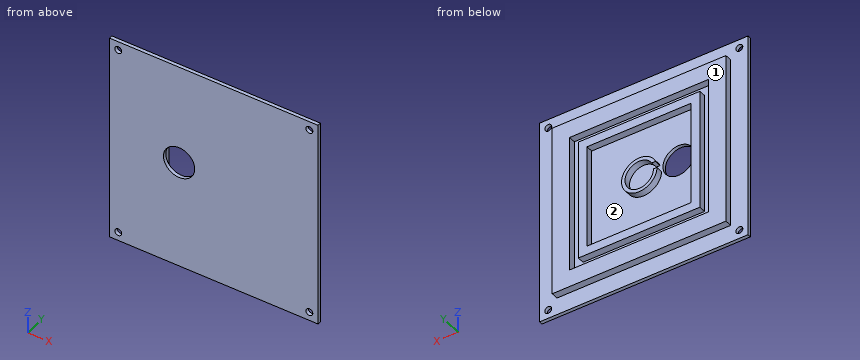
```python
from build123d import *

# Parameters (mm, degrees)
SKETCH1_W           = 152.4
SKETCH1_H           = 152.4
BOSS_EXTRUDE1_DEPTH = 2.54
SKETCH2_W           = 127
SKETCH2_H           = 127
BOSS_EXTRUDE3_DEPTH = 5.08
SKETCH3_W           = 101.6
SKETCH3_H           = 101.6
CUT_EXTRUDE2_DEPTH  = 5.08
SKETCH5_W           = 88.9
SKETCH5_H           = 88.9
BOSS_EXTRUDE4_DEPTH = 5.08
SKETCH6_W           = 76.2
SKETCH6_H           = 76.2
CUT_EXTRUDE3_DEPTH  = 5.08
BOSS_EXTRUDE5_DEPTH = 2.794
SKETCH8_R           = 11.43
CUT_EXTRUDE4_DEPTH  = 3.54
SKETCH9_R           = 2.54
CUT_EXTRUDE5_DEPTH  = 3.54
BOSS_EXTRUDE6_DEPTH = 4.9276


with BuildPart() as part:
    # Sketch1 → Boss-Extrude1 (new body)
    with BuildSketch(Plane(origin=(0, 0, 0), x_dir=(1, 0, 0), z_dir=(0, 1, 0))):
        Rectangle(SKETCH1_W, SKETCH1_H)
    extrude(amount=-BOSS_EXTRUDE1_DEPTH)

    # Sketch2 → Boss-Extrude3 (add)
    with BuildSketch(Plane(origin=(0, 0, 0), x_dir=(1, 0, 0), z_dir=(0, 1, 0))):
        Rectangle(SKETCH2_W, SKETCH2_H)
    extrude(amount=BOSS_EXTRUDE3_DEPTH)

    # Sketch3 → Cut-Extrude2 (cut)
    with BuildSketch(Plane(origin=(0, 5.08, 0), x_dir=(1, 0, 0), z_dir=(0, 1, 0))):
        Rectangle(SKETCH3_W, SKETCH3_H)
    extrude(amount=-CUT_EXTRUDE2_DEPTH, mode=Mode.SUBTRACT)

    # Sketch5 → Boss-Extrude4 (add)
    with BuildSketch(Plane(origin=(0, 0, 0), x_dir=(1, 0, 0), z_dir=(0, 1, 0))):
        Rectangle(SKETCH5_W, SKETCH5_H)
    extrude(amount=BOSS_EXTRUDE4_DEPTH)

    # Sketch6 → Cut-Extrude3 (cut)
    with BuildSketch(Plane(origin=(0, 5.08, 0), x_dir=(1, 0, 0), z_dir=(0, 1, 0))):
        Rectangle(SKETCH6_W, SKETCH6_H)
    extrude(amount=-CUT_EXTRUDE3_DEPTH, mode=Mode.SUBTRACT)

    # Sketch7 → Boss-Extrude5 (add)
    with BuildSketch(Plane(origin=(0, 0, 0), x_dir=(1, 0, 0), z_dir=(0, 1, 0))):
        with BuildLine():
            Line((-10.414, 0), (-12.954, 0))
            ThreePointArc((-12.954, 0), (12.691940102, 2.592445263), (-11.916363371, -5.08))
            Line((-11.916363371, -5.08), (-9.090929325, -5.08))
            ThreePointArc((-9.090929325, -5.08), (10.077805664, 2.624734082), (-10.414, 0))
        make_face()
    extrude(amount=BOSS_EXTRUDE5_DEPTH)

    # Sketch8 → Cut-Extrude4 (cut, through all)
    with BuildSketch(Plane(origin=(0, 0, 0), x_dir=(1, 0, 0), z_dir=(0, 1, 0))):
        with Locations((-25.4, -3.048)):
            Circle(SKETCH8_R)
    extrude(amount=-CUT_EXTRUDE4_DEPTH, mode=Mode.SUBTRACT)

    # Sketch9 → Cut-Extrude5 (cut, through all)
    with BuildSketch(Plane(origin=(0, 0, 0), x_dir=(1, 0, 0), z_dir=(0, 1, 0))):
        with Locations((-69.85, -69.85)):
            Circle(SKETCH9_R)
        with Locations((69.85, -69.85)):
            Circle(SKETCH9_R)
        with Locations((69.85, 69.85)):
            Circle(SKETCH9_R)
        with Locations((-69.85, 69.85)):
            Circle(SKETCH9_R)
    extrude(amount=-CUT_EXTRUDE5_DEPTH, mode=Mode.SUBTRACT)

    # Sketch7<2> → Boss-Extrude6 (add)
    with BuildSketch(Plane(origin=(0, 0, 0), x_dir=(1, 0, 0), z_dir=(0, 1, 0))):
        with BuildLine():
            Line((-10.414, 0), (-12.954, 0))
            ThreePointArc((-12.954, 0), (12.691940102, 2.592445263), (-11.916363371, -5.08))
            Line((-11.916363371, -5.08), (-9.090929325, -5.08))
            ThreePointArc((-9.090929325, -5.08), (10.077805664, 2.624734082), (-10.414, 0))
        make_face()
    extrude(amount=BOSS_EXTRUDE6_DEPTH)


solid = part.part
```
Model file for the job. Use its own axes, mm. Face numbers are marked on the shaded views. Coordinates: 2 decimals unless noted, no trailing zeros. Write each loop counter-clockwise with the first axis right and the second up, starting at its lowest first coordinate (ties: lowest second). Pieces come first, ordered by that corner, then holes. Notation, with made-up numbers: (-23, 67.5) - (4, 67.5) arc R22 cw to (4, 75.5) - close; hole circle Ø6 at (68, -25). An arc over 180 degrees is marked (long way). Use a Markdown table: item, result. Add a question column.
Item 1: Drill centre lines: line 1 along X through (y, z) = (2.5, -27.5); line 2 along Z through (x, y) = (69.85, -1.3). Where is each one in solid material? Low to high.
Item 2: Two-plate mould, pull along X, no slides. Class the marked faces 1 and 2: pulls with the +X half, pulls with the -X half, needs draft (parallel to the pull), parting line crosses it, or undercut.
Item 3: Band-saw the part on A-A, the plane y = 3. Write the cut outline in (x, z), and give its area (3 significant figures).
Item 4: Band-saw the part on C-C, the plane z = 69.85. Write the cut outline in (x, y).
Item 5: Band-saw the part on D-D, the plane x = 0. Write the cut outline in (y, z), and give its area (3 significant figures).
Item 6: Drop flat-ended pins along their axis: pin 1 (4 mm diameter, centred on x = 16, y = 3, fed in from -Z); pin 2 (1.5 mm diameter, centred on y = 3, z = -4.5, fed in from +X); pin 3 (2 mm diameter, centred on y = 1.5, z = 37.5, fed in from -X). Give the stop position or say it passes through.
Item 7: Band-saw the part on B-B, the plane x = 69.85. Write the cut outline in (y, z), and give its area (3 significant figures).
A:
| question | item | result |
|---|---|---|
| 1 | line 1 | x = -63.5 to -50.8, -44.45 to -38.1, 38.1 to 44.45, 50.8 to 63.5 |
| 1 | line 2 | z = -76.2 to -72.39, -67.31 to 67.31, 72.39 to 76.2 |
| 2 | face 1 | needs draft |
| 2 | face 2 | undercut |
| 3 | outline | (-63.5, -63.5) - (63.5, -63.5) - (63.5, 63.5) - (-63.5, 63.5) - close; (-44.45, -44.45) - (44.45, -44.45) - (44.45, 44.45) - (-44.45, 44.45) - close; (-12.95, 0) arc R12.95 ccw (long way) to (-11.92, 5.08) - (-9.09, 5.08) arc R10.41 cw (long way) to (-10.41, 0) - close; hole (-50.8, -50.8) - (50.8, -50.8) - (50.8, 50.8) - (-50.8, 50.8) - close; hole (-38.1, -38.1) - (38.1, -38.1) - (38.1, 38.1) - (-38.1, 38.1) - close |
| 3 | area | 8,080 mm² |
| 4 | outline | (-76.2, -2.54) - (-72.39, -2.54) - (-72.39, 0) - (-76.2, 0) - close; (-67.31, -2.54) - (67.31, -2.54) - (67.31, 0) - (-67.31, 0) - close; (72.39, -2.54) - (76.2, -2.54) - (76.2, 0) - (72.39, 0) - close |
| 5 | outline | (-2.54, -76.2) - (0, -76.2) - (0, -63.5) - (5.08, -63.5) - (5.08, -50.8) - (0, -50.8) - (0, -44.45) - (5.08, -44.45) - (5.08, -38.1) - (0, -38.1) - (0, -12.95) - (4.93, -12.95) - (4.93, -10.41) - (0, -10.41) - (0, 10.41) - (4.93, 10.41) - (4.93, 12.95) - (0, 12.95) - (0, 38.1) - (5.08, 38.1) - (5.08, 44.45) - (0, 44.45) - (0, 50.8) - (5.08, 50.8) - (5.08, 63.5) - (0, 63.5) - (0, 76.2) - (-2.54, 76.2) - close |
| 5 | area | 606 mm² |
| 6 | pin 1 | stops at z = -63.5 |
| 6 | pin 2 | stops at x = 63.5 |
| 6 | pin 3 | stops at x = -63.5 |
| 7 | outline | (-2.54, -76.2) - (0, -76.2) - (0, -72.39) - (-2.54, -72.39) - close; (-2.54, -67.31) - (0, -67.31) - (0, 67.31) - (-2.54, 67.31) - close; (-2.54, 72.39) - (0, 72.39) - (0, 76.2) - (-2.54, 76.2) - close |
| 7 | area | 361 mm² |
